from build123d import *

# Parameters (mm, degrees)
ESBO_O1_W                = 35
ESBO_O1_H                = 15
ESBO_O1_R                = 0.8
RESSALTO_EXTRUS_O1_DEPTH = 3
FILETE1_R                = 3


with BuildPart() as part:
    # Esboço1 → Ressalto-extrusão1 (new body)
    with BuildSketch(Plane(origin=(0, 0, 0), x_dir=(0, 0, -1), z_dir=(1, 0, 0))):
        Rectangle(ESBO_O1_W, ESBO_O1_H)
        with Locations((-14.5, 4.5)):
            Circle(ESBO_O1_R, mode=Mode.SUBTRACT)
        with Locations((14.5, -4.5)):
            Circle(ESBO_O1_R, mode=Mode.SUBTRACT)
    extrude(amount=RESSALTO_EXTRUS_O1_DEPTH)

    # Filete1
    filete1_edges = [part.edges().sort_by_distance(p)[0] for p in [
        (1.5, -7.5, -17.5),
        (1.5, -7.5, 17.5),
        (1.5, 7.5, 17.5),
        (1.5, 7.5, -17.5),
    ]]
    fillet(filete1_edges, radius=FILETE1_R)


solid = part.part
Source: CAD feature listing. Evaluate the final solid. Frame: model axes, mm. Round coordinates to 2 decimals unless told otherwise and drop trailing zeros. Write each loop counter-clockwise with the first axis right and the second up, starting at its lowest first coordinate (ties: lowest second). Pieces come first, ordered by that corner, then holes. Notation, with made-up numbers: (24.5, 2.5) - (45.5, 2.5) arc R11 cw to (45.5, 6.5) - close; hole circle Ø11 at (-29.5, 13.25). An arc over 180 degrees is marked (long way). Use CSV: the item, a comma, the result in double quotes. Start each with the question number.
(1) First-contact query: pin 1 Ø1.3 at (y, z) = (4.5, 14.5) entering from -X. Flat tip, straight axial feed; report the tip coordinate or a pass-through.
(2) Cut plane A-A, the plane x = 1.9. Return loops of the section in (y, z), and give its area (3 significant figures).
(3) Material intervals for probe 1 along Y at (x, z) = (1.35, -14.5); probe 2 along Y at (x, z) = (1.95, 14.5); probe 3 along Y at (x, z) = (0.6, 16), sorted ascending. Write a range as [from, to].
(4) Mould query, pull axis Z, two halves, no side actions, for faces 1 (the face through (3, 0, 0)), 2 (the face through (1.52, -6.64, -16.6)), 3 (the face through (1.48, 3.72, 14.67)), 4 (the face through (1.48, -4.99, -13.87)). Classes: pulls with the +Z half, pulls with the -Z half, needs draft (parallel to the pull), parting line crosses it, or undercut.
Geometry says:
1,pin 1,"through"
2,outline,"(-7.5, -14.5) arc R3 ccw to (-4.5, -17.5) - (4.5, -17.5) arc R3 ccw to (7.5, -14.5) - (7.5, 14.5) arc R3 ccw to (4.5, 17.5) - (-4.5, 17.5) arc R3 ccw to (-7.5, 14.5) - close; hole circle Ø1.6 at (-4.5, -14.5); hole circle Ø1.6 at (4.5, 14.5)"
2,area,"513 mm²"
3,probe 1,"[-7.5, -5.3], [-3.7, 7.5]"
3,probe 2,"[-7.5, 3.7], [5.3, 7.5]"
3,probe 3,"[-7.1, 7.1]"
4,face 1,"needs draft"
4,face 2,"pulls with the -Z half"
4,face 3,"undercut"
4,face 4,"undercut"
